The listing builds one solid part. Answer for the finished solid, in the listing's coordinates (mm). A direction names the side the tool comes from. Give positions to 0.01 mm unless a question says otherwise; leave off trailing zeros. Loops run counter-clockwise (first coordinate to the right, second up) from the corner with the lowest first, then second, coordinate; pieces in that order, holes last. Notation, with made-up numbers: M 88,-16.5 L 139,-16.5 A6 ccw 139,-5.5 Z; hole C -25.5,-10 d2. An arc over 180 degrees is marked long. Use one line per item in the form item = value. Start each with the question number.
1. The part is cut by section A-A (x = 48.5). Write down the section's boundary in (y, z), and give its area (3 significant figures).
2. Straight lines are drawn through the part: line 1 (X direction, y = -10.5, z = 3.35); line 2 (Y direction, x = 99.5, z = 2.6); line 3 (X direction, y = -11, z = 1.85). For each, find the intervals that lie inside material, in ascending order. Write a range as from..to.
3. The part is cut by section C-C (x = 146.5). Write down the section's boundary in (y, z), and give its area (3 significant figures).
4. The part is cut by section B-B (z = 2). Give the number of separate pieces and of enclosed holes in the cut face, and give its area (3 significant figures).
5. For faces 1 (the face through (55.664, 1.257, 1.972)), 2 (the face through (371.037, -0.64, 1.972)), determine the directions among +Z, -Z, +X, -X, +Y, -Y from which every point of the face is accessible in a straight line to the end or side of a thin tool.
6. Each of these flat-tipped pins is pushed along its axis until it touches: pin 1 Ø2 at (x, z) = (292.5, 2.5) entering from +Y; pin 2 Ø1 at (x, z) = (288, 3) entering from -Y. Where does it stop, or does it pass through?
7. The mould has two halves that part along Y. Classify faces 3 (the face through (122, 20, 4)), 4 (the face through (-2.548, -5.056, 1.972)), 5 (the face through (-31.45, 0.51, 1.97)): released by +Y, released by -Y, zero draft, split by the parting line, or undercut.
from build123d import *

# Parameters (mm, degrees)
SKETCH_1_R          = 5.03
SKETCH_1_R_2        = 9.53
SKETCH_1_R_3        = 2
EXTRUDE_1_DEPTH     = 4
CUT_EXTRUDE_1_DEPTH = 10


with BuildPart() as part:
    # 草图1 → 凸台-拉伸1 (new body)
    with BuildSketch(Plane.XY):
        with BuildLine():
            Line((348.542857143, 22.354285714), (71.15327348, 29.854285714))
            Line((71.15327348, 29.854285714), (-1.457142857, 29.854285714))
            ThreePointArc((-1.457142857, 29.854285714), (-31.457142857, -0.145714286), (-1.457142857, -30.145714286))
            Line((-1.457142857, -30.145714286), (348.542857143, -22.645714286))
            ThreePointArc((348.542857143, -22.645714286), (371.042857143, -0.145714286), (348.542857143, 22.354285714))
        make_face()
        with Locations((-1.457142857, -0.145714286)):
            Circle(SKETCH_1_R, mode=Mode.SUBTRACT)
        with Locations((348.542857143, -0.145714286)):
            Circle(SKETCH_1_R_2, mode=Mode.SUBTRACT)
        with Locations((-1.457142857, -25.145714286)):
            Circle(SKETCH_1_R_3, mode=Mode.SUBTRACT)
        with Locations((83.558658591, 24.490381358)):
            Circle(SKETCH_1_R_3, mode=Mode.SUBTRACT)
        with Locations((213.511166909, 20.976753342)):
            Circle(SKETCH_1_R_3, mode=Mode.SUBTRACT)
        with Locations(Location((228.490069199, -20.218274027, 0), (0, 0, 180))):
            Circle(SKETCH_1_R_3, mode=Mode.SUBTRACT)
        with Locations(Location((113.516463171, -22.681994157, 0), (0, 0, 180))):
            Circle(SKETCH_1_R_3, mode=Mode.SUBTRACT)
        with Locations((338.463675227, -17.754553898)):
            Circle(SKETCH_1_R_3, mode=Mode.SUBTRACT)
        with Locations((338.463675227, 17.463125327)):
            Circle(SKETCH_1_R_3, mode=Mode.SUBTRACT)
    extrude(amount=EXTRUDE_1_DEPTH)

    # 草图4 → 切除-拉伸1 (cut)
    with BuildSketch(Plane(origin=(0, 0, 0), x_dir=(-1, 0, 0), z_dir=(0, 0, -1))):
        with BuildLine():
            Line((-79.096608398, 14.937462311), (-31.566415003, -12.812828637))
            ThreePointArc((-31.566415003, -12.812828637), (-30.191694318, -16.218057795), (-33.143289006, -18.402899067))
            Line((-33.143289006, -18.402899067), (-97.422136429, -17.025495194))
            ThreePointArc((-97.422136429, -17.025495194), (-100.002344972, -15.442774062), (-99.890331665, -12.41788806))
            Line((-99.890331665, -12.41788806), (-83.141677637, 13.954999014))
            ThreePointArc((-83.141677637, 13.954999014), (-81.317264225, 15.261949688), (-79.096608398, 14.937462311))
        make_face()
        with BuildLine():
            Line((-116.768601629, -16.610928082), (-215.80395994, -14.488741833))
            ThreePointArc((-215.80395994, -14.488741833), (-218.215167386, -13.18412995), (-218.559093597, -10.464268138))
            Line((-218.559093597, -10.464268138), (-209.267574838, 15.089297949))
            Line((-209.267574838, 15.089297949), (-100.305174274, 18.035399938))
            ThreePointArc((-100.305174274, 18.035399938), (-97.614705316, 16.516735307), (-97.691624355, 13.428200228))
            Line((-97.691624355, 13.428200228), (-116.768601629, -16.610928082))
        make_face()
        with BuildLine():
            Line((-232.659749539, -14.127546341), (-285.953651799, -12.98553415))
            ThreePointArc((-285.953651799, -12.98553415), (-288.86244016, -10.38736889), (-286.746258648, -7.111199137))
            Line((-286.746258648, -7.111199137), (-228.938261452, 10.118012745))
            ThreePointArc((-228.938261452, 10.118012745), (-225.898326118, 9.300720915), (-225.261979027, 6.217826959))
            Line((-225.261979027, 6.217826959), (-232.659749539, -14.127546341))
        make_face()
        Polygon((-334.463675227, -5.68094836), (-281.386552555, 10.138264153), (-334.463675227, 8.703176307), align=None)
    extrude(amount=-CUT_EXTRUDE_1_DEPTH, mode=Mode.SUBTRACT)


solid = part.part
Derived:
q1.outline = M -29.08,0 L -18.07,0 L -18.07,4 L -29.08,4 Z; M -2.93,0 L 29.85,0 L 29.85,4 L -2.93,4 Z
q1.area = 175 mm2
q2.line_1 = -29.61..35.53, 98.67..112.89, 218.57..231.34, 288.85..368.52
q2.line_2 = -27.98..-16.13, -11.8..10.58, 17.95..29.09
q2.line_3 = -29.42..34.67, 98.99..113.21, 218.7..231.52, 288.71..368.25
q3.outline = M -26.98,0 L -15.97,0 L -15.97,4 L -26.98,4 Z; M 16.79,0 L 27.82,0 L 27.82,4 L 16.79,4 Z
q3.area = 88.1 mm2
q4.separate_pieces = 1
q4.enclosed_holes = 13
q4.area = 14,300 mm2
q5.face_1 = +Z, -Z
q5.face_2 = +Z, -Z, +X
q6.pin_1 = 23.9
q6.pin_2 = -23.95
q7.face_3 = zero draft
q7.face_4 = undercut
q7.face_5 = split by the parting line
